from build123d import *

# Parameters (mm, degrees)
BOSS_EXTRUDE1_DEPTH      = 7
BOSS_EXTRUDE1_DEPTH_BACK = 7
SKETCH3_R                = 7
BOSS_EXTRUDE2_DEPTH      = 3
CUT_EXTRUDE1_DEPTH       = 23
CUT_EXTRUDE1_DEPTH_BACK  = 23
SKETCH4_R                = 2.6
BOSS_EXTRUDE3_DEPTH      = 3
CUT_EXTRUDE2_DEPTH       = 20
CUT_EXTRUDE2_DEPTH_BACK  = 30
SKETCH6_W                = 36.146068324
SKETCH6_H                = 79.881394618
SKETCH7_W                = 6
SKETCH7_H                = 2
BOSS_EXTRUDE4_DEPTH      = 25
SKETCH8_R                = 1.5
CUT_EXTRUDE3_DEPTH       = 23
SKETCH9_W                = 6
SKETCH9_H                = 2
BOSS_EXTRUDE5_DEPTH      = 11
SKETCH10_W               = 10.612588882
SKETCH10_H               = 43.057143259
CUT_EXTRUDE4_DEPTH       = 10
CUT_EXTRUDE5_DEPTH       = 22
BOSS_EXTRUDE6_DEPTH      = 1.5
SKETCH17_W               = 50
SKETCH17_H               = 12
CUT_EXTRUDE7_DEPTH       = 22
SKETCH18_W               = 7
SKETCH18_H               = 4
CUT_EXTRUDE8_DEPTH       = 22


with BuildPart() as part:
    # Sketch2 → Boss-Extrude1 (new, two sides: drawn at the far end of the back side and taken through both)
    with BuildSketch(Plane(origin=(0, 0, 0), x_dir=(1, 0, 0), z_dir=(0, 1, 0)).offset(-BOSS_EXTRUDE1_DEPTH_BACK)):
        Polygon((12, 30), (12, -30), (9, -30), (9, -1.5), (-9, -1.5), (-9, -30), (-12, -30), (-12, 30), (-9, 30), (-9, 1.5), (9, 1.5), (9, 30), align=None)
    extrude(amount=BOSS_EXTRUDE1_DEPTH + BOSS_EXTRUDE1_DEPTH_BACK)

    # Sketch3 → Boss-Extrude2 (add)
    with BuildSketch(Plane(origin=(12, 0, 0), x_dir=(0, 0, -1), z_dir=(1, 0, 0))):
        with Locations((-30, 0)):
            Circle(SKETCH3_R)
        with Locations((30, 0)):
            Circle(SKETCH3_R)
    boss_extrude2 = extrude(amount=-BOSS_EXTRUDE2_DEPTH)

    # Mirror1: Boss-Extrude2 across plane
    add(boss_extrude2.mirror(Plane.ZY))

    # Sketch4 → Cut-Extrude1 (cut, two sides: drawn at the far end of the back side and taken through both)
    with BuildSketch(Plane.ZY.offset(-CUT_EXTRUDE1_DEPTH_BACK)):
        with Locations(Location((-30, 0, 0), (0, 0, 180))):
            Circle(SKETCH4_R)
        with Locations(Location((30, 0, 0), (0, 0, 180))):
            Circle(SKETCH4_R)
    extrude(amount=CUT_EXTRUDE1_DEPTH + CUT_EXTRUDE1_DEPTH_BACK, mode=Mode.SUBTRACT)

    # Sketch5 → Boss-Extrude3 (add)
    with BuildSketch(Plane.ZY.offset(12)):
        Polygon((-30, 7), (-24.155374342, 13.339180653), (-3.984430585, 16.782248387), (-3.984430585, 13.558363221), (-6.564031008, 12.252853794), (-9.961076462, 7), align=None)
        Polygon((5.630173652, 7), (6.872920148, 8.921659787), (16.024340395, 8.921659787), (16.024340395, 11.520201473), (23.010764714, 11.520201473), (24.017423371, 9.614604237), (26.442728945, 9.614604237), (25.802127981, 10.827257024), (33.625376893, 10.827257024), (39.584451678, 2.208760433), (39.584451678, -0.649635421), (35.450408088, -0.649635421), (35.450408088, 3.248177107), (30.561687085, 6.409736158), (5.630173652, 6.409736158), align=None)
        Polygon((-30, -7), (-17.229678236, -13.21512033), (-6.200995871, -13.21512033), (-6.200995871, -8.829973728), (-9.961076462, -7), align=None)
        Polygon((9.961076462, -7), (15.524820582, -9.707789187), (15.524820582, -13.295871625), (32.135298846, -13.295871625), (32.135298846, -11.501830406), (39.584451678, -7), (39.584451678, -3.334795163), (35.450408088, -3.334795163), (31.744983073, -5.574136385), (9.961076462, -5.574136385), align=None)
    boss_extrude3 = extrude(amount=-BOSS_EXTRUDE3_DEPTH)

    # Mirror2: Boss-Extrude3 across plane
    add(boss_extrude3.mirror(Plane.ZY))

    # Sketch6 → Cut-Extrude2 (cut, two sides: drawn at the far end of the back side and taken through both)
    with BuildSketch(Plane(origin=(0, 7, 0), x_dir=(1, 0, 0), z_dir=(0, 1, 0)).offset(-CUT_EXTRUDE2_DEPTH_BACK)):
        with Locations((9.073034162, -2.940697309)):
            Rectangle(SKETCH6_W, SKETCH6_H)
    extrude(amount=CUT_EXTRUDE2_DEPTH + CUT_EXTRUDE2_DEPTH_BACK, mode=Mode.SUBTRACT)

    # Sketch7 → Boss-Extrude4 (add)
    with BuildSketch(Plane(origin=(-9, 0, 0), x_dir=(0, 0, -1), z_dir=(1, 0, 0))):
        Rectangle(SKETCH7_W, SKETCH7_H)
    extrude(amount=BOSS_EXTRUDE4_DEPTH)

    # Sketch8 → Cut-Extrude3 (cut)
    with BuildSketch(Plane(origin=(0, 1, 0), x_dir=(1, 0, 0), z_dir=(0, 1, 0))):
        with Locations(Location((13, 0, 0), (0, 0, 270))):
            Circle(SKETCH8_R)
        with Locations(Location((5, 0, 0), (0, 0, 270))):
            Circle(SKETCH8_R)
    extrude(amount=-CUT_EXTRUDE3_DEPTH, mode=Mode.SUBTRACT)

    # Sketch9 → Boss-Extrude5 (add)
    with BuildSketch(Plane(origin=(-9, 0, 0), x_dir=(0, 0, -1), z_dir=(1, 0, 0))):
        with Locations((0, -2)):
            Rectangle(SKETCH9_W, SKETCH9_H)
    extrude(amount=BOSS_EXTRUDE5_DEPTH)

    # Sketch10 → Cut-Extrude4 (cut)
    with BuildSketch(Plane(origin=(-9, 0, 0), x_dir=(0, 0, -1), z_dir=(1, 0, 0))):
        with Locations((-43.306294441, -0.681634791)):
            Rectangle(SKETCH10_W, SKETCH10_H)
    extrude(amount=-CUT_EXTRUDE4_DEPTH, mode=Mode.SUBTRACT)

    # Sketch11 → Cut-Extrude5 (cut)
    with BuildSketch(Plane.ZY):
        Polygon((39.991694919, -1.896890181), (29.115063305, 13.833775376), (39.991694919, 13.833775376), align=None)
    extrude(amount=CUT_EXTRUDE5_DEPTH, mode=Mode.SUBTRACT)

    # Sketch12 → Boss-Extrude6 (add)
    with BuildSketch(Plane.ZY.offset(12)):
        with BuildLine():
            Line((-29.251939175, 5.448890254), (-13.9, 4.4))
            ThreePointArc((-13.9, 4.4), (-9.5, 0), (-13.9, -4.4))
            Line((-13.9, -4.4), (-29.251939175, -5.448890254))
            ThreePointArc((-29.251939175, -5.448890254), (-35.5, 0), (-29.251939175, 5.448890254))
        make_face()
        with BuildLine():
            Line((29.251939175, -5.448890254), (13.9, -4.4))
            ThreePointArc((13.9, -4.4), (9.5, 0), (13.9, 4.4))
            Line((13.9, 4.4), (29.251939175, 5.448890254))
            ThreePointArc((29.251939175, 5.448890254), (35.5, 0), (29.251939175, -5.448890254))
        make_face()
    extrude(amount=BOSS_EXTRUDE6_DEPTH)

    # Sketch17 → Cut-Extrude7 (cut)
    with BuildSketch(Plane(origin=(0, 1, 0), x_dir=(1, 0, 0), z_dir=(0, 1, 0))):
        with Locations((16, 3)):
            Rectangle(SKETCH17_W, SKETCH17_H)
    extrude(amount=-CUT_EXTRUDE7_DEPTH, mode=Mode.SUBTRACT)

    # Sketch18 → Cut-Extrude8 (cut)
    with BuildSketch(Plane(origin=(-9, 0, 0), x_dir=(0, 0, -1), z_dir=(1, 0, 0))):
        Rectangle(SKETCH18_W, SKETCH18_H)
    extrude(amount=-CUT_EXTRUDE8_DEPTH, mode=Mode.SUBTRACT)


solid = part.part
Geometry: final body of the model. Coordinates: model frame, mm. A direction names the side the tool comes from. Give positions to 0.01 mm unless a question says otherwise; leave off trailing zeros. Order: outer loops, then holes, each group sorted by start corner. A loop starts at its lowest first (then second) coordinate and runs counter-clockwise, first axis right, second up. Notation, with made-up numbers: (39.5, -9.75) - (83.5, -9.75) arc R23 cw to (83.5, 29.25) - close; hole circle Ø3 at (32, 11.25). An arc over 180 degrees is marked (long way). Use CSV: the item, a comma, the result in double quotes.
1. Section query A-A (y = 0). Output: boundary loops of the cut face in (x, z), plus the area to 3 significant figures.
Answers below:
outline,"(-13.5, -35.5) - (-12, -35.5) - (-12, -37) - (-9, -37) - (-9, -32.6) - (-12, -32.6) - (-12, -27.4) - (-9, -27.4) - (-9, -3.5) - (-12, -3.5) - (-12, -9.5) - (-13.5, -9.5) - close; (-13.5, 9.5) - (-12, 9.5) - (-12, 3.5) - (-9, 3.5) - (-9, 27.4) - (-12, 27.4) - (-12, 32.6) - (-9, 32.6) - (-9, 38) - (-12, 38) - (-12, 35.5) - (-13.5, 35.5) - close"
area,"251 mm2"
2. Section query B-B (z = 30). Output: boundary loops of the cut face in (x, y), plus the area to 3 significant figures.
Answers below:
outline,"(-13.5, -5.5) - (-12, -5.5) - (-12, -13.3) - (-9, -13.3) - (-9, -2.6) - (-12, -2.6) - (-12, 2.6) - (-9, 2.6) - (-9, 10.83) - (-12, 10.83) - (-12, 5.5) - (-13.5, 5.5) - close"
area,"73.3 mm2"
3. Section query C-C (x = -10.25). Give the number of separate pieces and of enclosed holes in the cut face, plus the area to 3 significant figures.
Answers below:
separate pieces,"1"
enclosed holes,"3"
area,"1,420 mm2"
4. Contact query for flat-ended pins moving along their axis: pin 1 (0.9 mm diameter, centred on x = -10.5, z = 11.5, fed in from +Y); pin 2 (2 mm diameter, centred on x = -11, z = -2, fed in from +Y); pin 3 (0.9 mm diameter, centred on x = -10, z = -5, fed in from -Y); pin 4 (15 mm diameter, centred on y = 8, z = 6.5, fed in from -X). Output: stop coordinate, or through.
Answers below:
pin 1,"y = 8.92"
pin 2,"y = 7"
pin 3,"y = -7"
pin 4,"x = -13.5"
5. Section query D-D (z = -19). Output: boundary loops of the cut face in (x, y), plus the area to 3 significant figures.
Answers below:
outline,"(-13.5, -4.75) - (-12, -4.75) - (-12, -12.35) - (-9, -12.35) - (-9, 14.22) - (-12, 14.22) - (-12, 4.75) - (-13.5, 4.75) - close"
area,"94.0 mm2"
6. Mould query, pull axis Y, two halves, no side actions, for faces 5 (the face through (-10.521, 10.125, -27.119)), 6 (the face through (-11, -12, 32.135)), 7 (the face through (-10, -2, 0)). Classes: +Y half, -Y half, draft (parallel to the pull), parting line (faces both ways), or undercut.
Answers below:
face 5,"+Y half"
face 6,"draft"
face 7,"undercut"
7. Access query for faces 1 (the face through (-12.7, -0.1, 9.5)), 2 (the face through (-10.5, -0.1, 32.6)), 3 (the face through (-11, 10, 16.024)), 4 (the face through (-12.74, -4.93, 21.68)). Directions: +Z, -Z, +X, -X, +Y, -Y. A direction counts if a zero-diameter tool reaches every point of the face in a straight line with its end or side. Return the directions, or none.
Answers below:
face 1,"-X"
face 2,"+X"
face 3,"+X, -X, +Y"
face 4,"-X, -Y"
8. Material intervals for line 1 along Y through (x, z) = (-10.95, 30); line 2 along Y through (x, z) = (-10.25, -30); line 3 along Z through (x, y) = (-10.45, 0.5), sorted ascending. Write a range as from..to.
Answers below:
line 1,"-13.3..-2.6, 2.6..10.83"
line 2,"-7..-2.6, 2.6..7"
line 3,"-36.98..-32.55, -27.45..-3.5, 3.5..27.45, 32.55..38"
